Study the drawing (mm; zero at the part's minimum x, y, z) and answer. Coordinates: 2 decimals unless noted, no trailing zeros. Loops run counter-clockwise (first coordinate to the right, second up) from the corner with the lowest first, then second, coordinate; pieces in that order, holes last. Notation, with made-up numbers: (43, 4) -> (78, 4) arc R17 ccw to (78, 15) -> close; hole circle Ø9 at (34.25, 85). An arc over 180 degrees is marked (long way). Answer as a JSON object with one key per item and string values. Group by question number.
Q1. The part is cut by section C-C on z = 1.8. Write down the section's boundary in (x, y), and give its area (3 significant figures).
Q2. Straight lines are drawn through the part: line 1 along Y through (x, z) = (6.75, 0.75); line 2 along X through (y, z) = (14, 2.8) (1 decimal); line 3 along X through (y, z) = (13, 2.35) (1 decimal). For each, find the intervals that lie inside material, in ascending order. Write a range as [from, to].
Q3. The part is cut by section B-B on x = 6. Write down the section's boundary in (y, z).
Q4. Determine the mould class of the marked faces 1, 2 and 3 for opening direction X: released by +X, released by -X, zero draft, split by the parting line, or undercut.
Q5. Each of these flat-tipped pins is pushed along its axis until it touches: P1, Ø2, axis at y = 3, z = 3, coming from the -X side; P2, Ø1.3, axis at x = 6.58, y = 15, coming from the +Z side; P3, Ø1.5, axis at y = 15, z = 2.5, coming from the +X side. Where does it stop, or does it pass through?
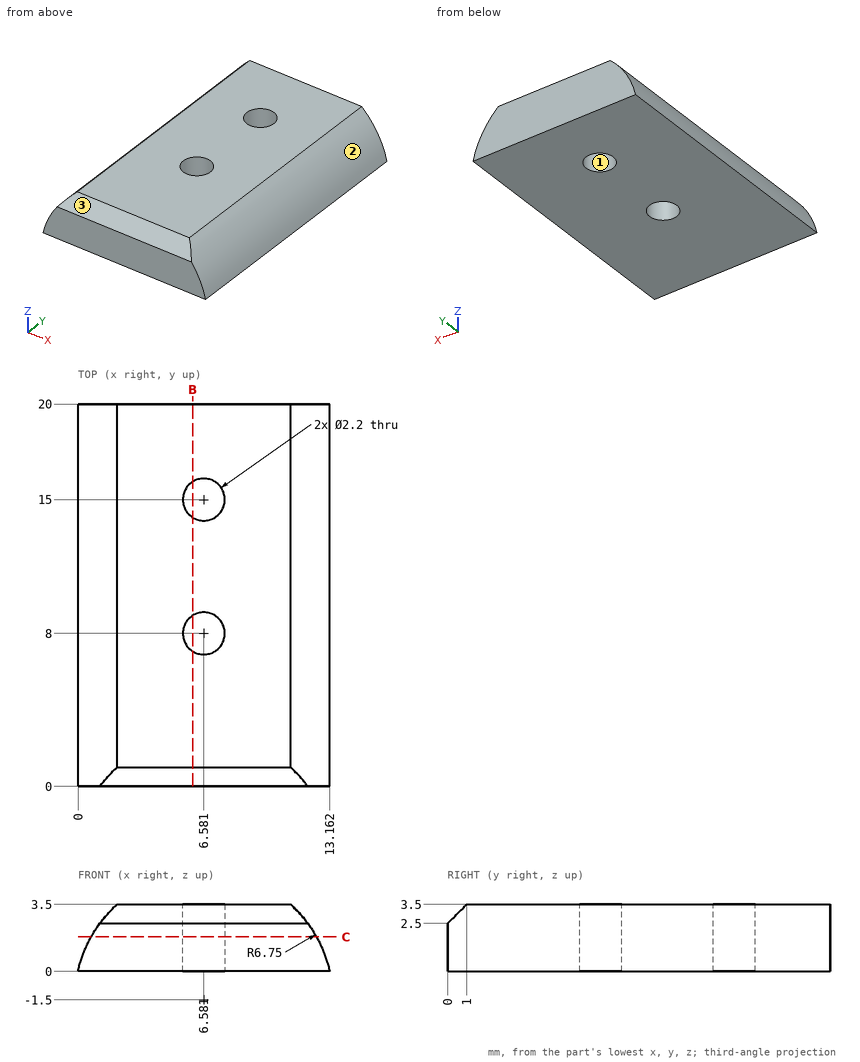
Final values:
{
 "1": {"outline": "(0.69, 0) -> (12.47, 0) -> (12.47, 20) -> (0.69, 20) -> close; hole circle Ø2.2 at (6.58, 8); hole circle Ø2.2 at (6.58, 15)", "area": "228 mm2"},
 "2": {"line 1": "y = [0, 6.91], [9.09, 13.91], [16.09, 20]", "line 2": "x = [1.4, 6.1], [7, 11.8]", "line 3": "x = [1, 12.1]"},
 "3": {"outline": "(0, 0) -> (7.07, 0) -> (7.07, 3.5) -> (1, 3.5) -> (0, 2.5) -> close; (8.93, 0) -> (14.07, 0) -> (14.07, 3.5) -> (8.93, 3.5) -> close; (15.93, 0) -> (20, 0) -> (20, 3.5) -> (15.93, 3.5) -> close"},
 "4": {"face 1": "undercut", "face 2": "released by +X", "face 3": "zero draft"},
 "5": {"P1": "stops at x = 0.81", "P2": "passes through", "P3": "stops at x = 12.5"}
}
